For this review, take the finished solid that the model builds, in its own axes (mm). Face numbers are marked on the shaded views. A direction names the side the tool comes from. Give positions to 0.01 mm unless a question says otherwise; leave off trailing zeros. Order: outer loops, then holes, each group sorted by start corner. A loop starts at its lowest first (then second) coordinate and runs counter-clockwise, first axis right, second up. Notation, with made-up numbers: (10, 42) - (27, 42) arc R31 ccw to (27, 73) - close; hole circle Ø9 at (14.5, 79.5). An arc over 180 degrees is marked (long way). One line per item, written item: value.
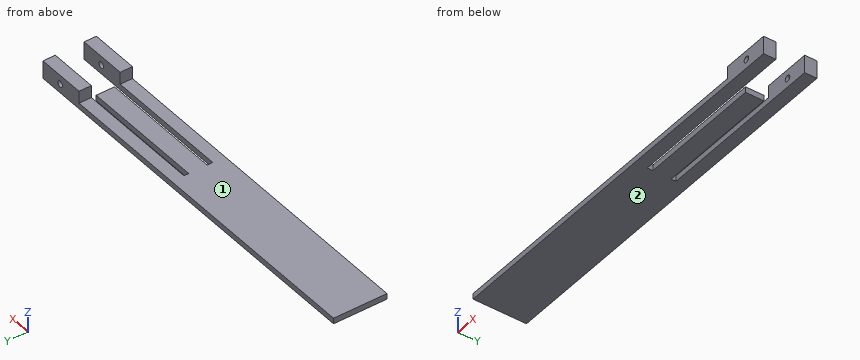
```python
from build123d import *

# Parameters (mm, degrees)
F1_DEPTH = 2.8
F2_DEPTH = 42.8
F3_DEPTH = 1.439
F4_DEPTH = 85.376
F5_W     = 23.89
F5_H     = 6.0450145833
F5_H_2   = 6.0446187854
F6_DEPTH = 6
F7_R     = 1.5
F8_DEPTH = 27.5
F9_DEPTH = 23.89


with BuildPart() as f1:
    # F0 (on Top) → F1 (new body)
    with BuildSketch(Plane.XY):
        Polygon((-75.0034600496, -12.3867541552), (75.0034600496, -12.3867541552), (75.0034600496, -6.3421353698), (-10.3727839887, -6.3421353698), (-10.3727839887, -3.5960208625), (75.0034600496, -3.5960208625), (75.0034600496, 5.426927004), (-10.3727839887, 5.426927004), (-10.3727839887, 7.7807395719), (75.0034600496, 7.7807395719), (75.0034600496, 12.3867541552), (-75.0034600496, 12.3867541552), align=None)
    extrude(amount=F1_DEPTH)

    # F2 (add): a face of the model
    f2_faces = [f1.faces().sort_by_distance(p)[0] for p in [
        (-75.0034600496, 0, 1.4),
    ]]
    extrude(f2_faces, amount=F2_DEPTH)

    # F3 (add): a face of the model
    f3_faces = [f1.faces().sort_by_distance(p)[0] for p in [
        (-21.4, 12.3867541552, 1.4),
    ]]
    extrude(f3_faces, amount=F3_DEPTH)

    # F4 (cut): a face of the model
    f4_faces = [f1.faces().sort_by_distance(p)[0] for p in [
        (-21.4, 13.8257541552, 1.4),
    ]]
    extrude(f4_faces, amount=F4_DEPTH, mode=Mode.SUBTRACT)

    # F5 (on face) → F6 (join)
    with BuildSketch(Plane.XY.offset(2.8)):
        with Locations((63.0584600496, 10.8032468635)):
            Rectangle(F5_W, F5_H)
        with Locations((63.0584600496, -9.3644447625)):
            Rectangle(F5_W, F5_H_2)
    extrude(amount=F6_DEPTH)

    # F7 (on face) → F8 (cut)
    with BuildSketch(Plane.XZ.offset(12.3867541552)):
        with Locations((63.6097000496, 4.4)):
            Circle(F7_R)
    extrude(amount=-F8_DEPTH, mode=Mode.SUBTRACT)

    # F9 (cut): a face of the model
    f9_faces = [f1.faces().sort_by_distance(p)[0] for p in [
        (75.0034600496, 0.9154530708, 1.4),
    ]]
    extrude(f9_faces, amount=-F9_DEPTH, mode=Mode.SUBTRACT)


solid = f1.part
```
(1) For P1, Ø2, axis at x = 33.5, z = 5.5, coming from the +Y side; P2, Ø8, axis at x = 6.5, y = 6, coming from the +Z side; P3, Ø3, axis at y = 10.5, z = 4.5, coming from the -X side; P4, Ø4, axis at y = 9, z = 4, coming from the -X side, all flat-tipped, find the tip position at first contact; note any pin that passes through.
Answers below:
P1: passes through
P2: stops at z = 2.8
P3: stops at x = 51.11
P4: stops at x = -117.8
(2) Take a section at B-B (z = 4.4). Write out the cut boundary in (x, y), then the cut area to 3 significant figures.
Answers below:
outline: (51.11, -12.39) - (62.11, -12.39) - (62.11, -6.34) - (51.11, -6.34) - close; (51.11, 7.78) - (62.11, 7.78) - (62.11, 13.83) - (51.11, 13.83) - close; (65.11, -12.39) - (75, -12.39) - (75, -6.34) - (65.11, -6.34) - close; (65.11, 7.78) - (75, 7.78) - (75, 13.83) - (65.11, 13.83) - close
area: 253 mm^2
(3) Wall thickness on line 1 (Y direction, x = 59, z = 8); line 2 (Z direction, x = -16, y = -3.25); line 3 (X direction, y = 11.5, z = 6.25): over which ranges is each line inside the solid? List them lowest first. Write a range as from..to.
Answers below:
line 1: y = -12.39..-6.34, 7.78..13.83
line 2: z = 0..2.8
line 3: x = 51.11..75
(4) Take a section at C-C (y = 3.5). Write out the cut boundary in (x, z), then the cut area to 3 significant figures.
Answers below:
outline: (-117.8, 0) - (51.11, 0) - (51.11, 2.8) - (-117.8, 2.8) - close
area: 473 mm^2
(5) Take a section at D-D (x = -36). Write out the cut boundary in (y, z).
Answers below:
outline: (-12.39, 0) - (13.83, 0) - (13.83, 2.8) - (-12.39, 2.8) - close
(6) Machinability: for the marked faces 1 and 2, which of the approach directions +Z, -Z, +X, -X, +Y, -Y give a long, thin tool a straight path to every point of the face, cutting with its end or side? Answer none if there is none.
Answers below:
face 1: +Z, -X, +Y, -Y
face 2: -Z, +X, -X, +Y, -Y
(7) Take a section at A-A (x = 44.5). Write out the cut boundary in (y, z), then the cut area to 3 significant figures.
Answers below:
outline: (-12.39, 0) - (-6.34, 0) - (-6.34, 2.8) - (-12.39, 2.8) - close; (-3.6, 0) - (5.43, 0) - (5.43, 2.8) - (-3.6, 2.8) - close; (7.78, 0) - (13.83, 0) - (13.83, 2.8) - (7.78, 2.8) - close
area: 59.1 mm^2
